from build123d import *

# Parameters (mm, degrees)
SKETCH1_W           = 39.8
SKETCH1_H           = 19.8
BOSS_EXTRUDE1_DEPTH = 1.6
SKETCH2_R           = 1.9
BOSS_EXTRUDE2_DEPTH = 1.6
SKETCH3_R           = 1
SKETCH3_R_2         = 2.1
CUT_EXTRUDE1_DEPTH  = 1.6
SKETCH4_W           = 4.3
SKETCH4_H           = 6
BOSS_EXTRUDE3_DEPTH = 6
SKETCH5_W           = 5
SKETCH5_H           = 10
BOSS_EXTRUDE4_DEPTH = 8


with BuildPart() as part:
    # Sketch1 → Boss-Extrude1 (new body)
    with BuildSketch(Plane(origin=(0, 0, 0), x_dir=(1, 0, 0), z_dir=(0, 1, 0))):
        Rectangle(SKETCH1_W, SKETCH1_H)
    extrude(amount=BOSS_EXTRUDE1_DEPTH)

    # Sketch2 → Boss-Extrude2 (add)
    with BuildSketch(Plane(origin=(0, 0, 0), x_dir=(1, 0, 0), z_dir=(0, 1, 0))):
        with Locations((-10, 10)):
            Circle(SKETCH2_R)
        with Locations((20, 0)):
            Circle(SKETCH2_R)
        with Locations((-10, -10)):
            Circle(SKETCH2_R)
    extrude(amount=BOSS_EXTRUDE2_DEPTH)

    # Sketch3 → Cut-Extrude1 (cut)
    with BuildSketch(Plane(origin=(0, 1.6, 0), x_dir=(1, 0, 0), z_dir=(0, 1, 0))):
        with Locations(Location((-10, 10, 0), (0, 0, 270))):
            Circle(SKETCH3_R)
        with Locations(Location((-10, -10, 0), (0, 0, 270))):
            Circle(SKETCH3_R)
        with Locations(Location((20, 0, 0), (0, 0, 270))):
            Circle(SKETCH3_R)
        with Locations((10, 10)):
            Circle(SKETCH3_R_2)
        with Locations((10, -10)):
            Circle(SKETCH3_R_2)
        with Locations((-20, 0)):
            Circle(SKETCH3_R_2)
    extrude(amount=-CUT_EXTRUDE1_DEPTH, mode=Mode.SUBTRACT)

    # Sketch4 → Boss-Extrude3 (add)
    with BuildSketch(Plane(origin=(0, 1.6, 0), x_dir=(1, 0, 0), z_dir=(0, 1, 0))):
        with Locations((16.55, 0)):
            Rectangle(SKETCH4_W, SKETCH4_H)
    extrude(amount=BOSS_EXTRUDE3_DEPTH)

    # Sketch5 → Boss-Extrude4 (add)
    with BuildSketch(Plane(origin=(0, 1.6, 0), x_dir=(1, 0, 0), z_dir=(0, 1, 0))):
        with Locations((-16.2, 0)):
            Rectangle(SKETCH5_W, SKETCH5_H)
    extrude(amount=BOSS_EXTRUDE4_DEPTH)


solid = part.part
Geometry: final body of the model. Coordinates: model frame, mm. A direction names the side the tool comes from. Round coordinates to 2 decimals unless told otherwise and drop trailing zeros. Order: outer loops, then holes, each group sorted by start corner. A loop starts at its lowest first (then second) coordinate and runs counter-clockwise, first axis right, second up.
Q1. Material intervals for probe 1 along X at (y, z) = (0.8, -10); probe 2 along X at (y, z) = (7.25, 0.75); probe 3 along Y at (x, z) = (-2, 5), sorted ascending.
Result sheet:
probe 1: x = -11.9 to -11, -9 to -8.1
probe 2: x = -18.7 to -13.7, 14.4 to 18.7
probe 3: y = 0 to 1.6
Q2. Section A-A, the plane z = 0. Output: boundary loops of the cut face in (x, y), and give its area (3 significant figures).
Result sheet:
outline: (-18.7, 1.6) - (-17.9, 1.6) - (-17.9, 0) - (19, 0) - (19, 1.6) - (18.7, 1.6) - (18.7, 7.6) - (14.4, 7.6) - (14.4, 1.6) - (-13.7, 1.6) - (-13.7, 9.6) - (-18.7, 9.6) - close; (21, 0) - (21.9, 0) - (21.9, 1.6) - (21, 1.6) - close
area: 126 mm2
Q3. Section D-D, the plane x = 10. Output: boundary loops of the cut face in (y, z).
Result sheet:
outline: (0, -7.9) - (1.6, -7.9) - (1.6, 7.9) - (0, 7.9) - close
Q4. Pin query (flat end, axial travel): pin 1 (1.6 mm diameter, centred on x = 20, z = 0, fed in from +Y); pin 2 (1.3 mm diameter, centred on x = 17.5, z = -1, fed in from +Y); pin 3 (3.5 mm diameter, centred on x = 16.5, y = 3.5, fed in from +Z); pin 4 (0.5 mm diameter, centred on x = 15, y = 1, fed in from +Z). Return the tip coordinate at first contact, or that it passes through.
Result sheet:
pin 1: passes through
pin 2: stops at y = 7.6
pin 3: stops at z = 3
pin 4: stops at z = 9.9
Q5. Section B-B, the plane x = -10. Output: boundary loops of the cut face in (y, z), and give its area (3 significant figures).
Result sheet:
outline: (0, -11.9) - (1.6, -11.9) - (1.6, -11) - (0, -11) - close; (0, -9) - (1.6, -9) - (1.6, 9) - (0, 9) - close; (0, 11) - (1.6, 11) - (1.6, 11.9) - (0, 11.9) - close
area: 31.7 mm2
Q6. Mould query, pull axis X, two halves, no side actions, for faces 1 (the face through (-19.9, 1, -6)), 2 (the face through (-16, 6, 5)), 3 (the face through (10, 0.8, -7.9)). Classes: released by +X, released by -X, zero draft, split by the parting line, or undercut.
Result sheet:
face 1: released by -X
face 2: zero draft
face 3: undercut
Q7. Section C-C, the plane z = -7.5. Output: boundary loops of the cut face in (x, y).
Result sheet:
outline: (-19.9, 0) - (19.9, 0) - (19.9, 1.6) - (-19.9, 1.6) - close
Q8. Access query for faces 4 (the face through (19.9, 1, 6)), 5 (the face through (-18.7, 6, 0)), 6 (the face through (17, 5, 3)), 7 (the face through (19.9, 1, -6)). Directions: +Z, -Z, +X, -X, +Y, -Y. A direction counts if a zero-diameter tool reaches every point of the face in a straight line with its end or side. Return the directions, or none.
Result sheet:
face 4: +Z, +X, +Y, -Y
face 5: +Z, -Z, -X, +Y
face 6: +Z, +X, +Y
face 7: -Z, +X, +Y, -Y
